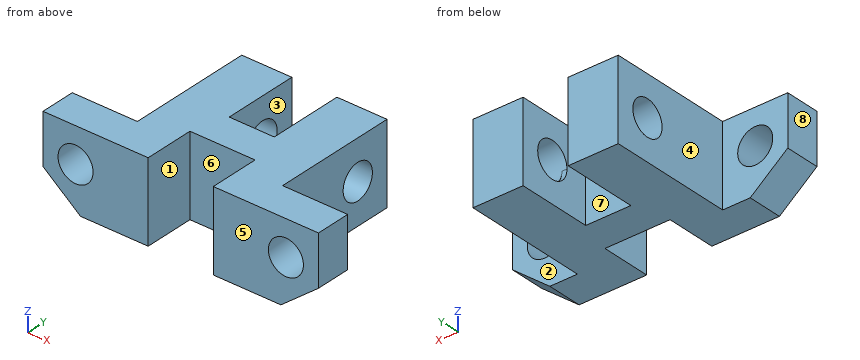
Autodesk Fusion 360 part; units mm, degrees
sketch "Boceto1" plane through (0, 0, 0) normal (0, 0, 1) x (1, 0, 0)
  line L0 (0, 0) -> (4.5, 0)
  line L1 (4.5, 0) -> (4.5, 15)
  line L2 (4.5, 15) -> (14.5, 15)
  line L3 (14.5, 15) -> (14.5, -10)
  line L4 (14.5, -10) -> (27.5, -10)
  line L5 (27.5, -10) -> (27.5, -17)
  line L6 (0, -7) -> (6.5, -7)
  line L7 (6.5, -7) -> (6.5, -17)
  line L8 (6.5, -17) -> (27.5, -17)
  line L9 (0, -7) -> (-6.5, -7)
  line L10 (-27.5, -10) -> (-27.5, -17)
  line L11 (-6.5, -7) -> (-6.5, -17)
  line L12 (-6.5, -17) -> (-27.5, -17)
  line L13 (-14.5, -10) -> (-27.5, -10)
  line L14 (-4.5, 0) -> (-4.5, 15)
  line L15 (-14.5, 15) -> (-14.5, -10)
  line L16 (0, 0) -> (-4.5, 0)
  line L17 (-4.5, 15) -> (-14.5, 15)
  dimension "d1" = 4.5
  dimension "d2" = 15
  dimension "d3" = 10
  dimension "d4" = 25
  dimension "d5" = 13
  dimension "d6" = 7
  dimension "d7" = 6.5
  dimension "d8" = 7
  dimension "d9" = 32
extrude "Extruir1" add sketch "Boceto1" along normal blind 16
sketch "Boceto2" plane through (0, 0, 0) normal (1, 0, 0) x (0, 1, 0)
  circle A0 centre (8, 8.0871) radius 3.5
  line L0 (15, 0) -> (15, 16)
  dimension "d12" = 7
  dimension "d13" = 7
sketch "Boceto3" plane through (-14.5, 0, 0) normal (-1, 0, 0) x (0, -1, 0)
  line L0 (-15, 0) -> (10, 0)
  line L1 (10, 0) -> (10, 16)
  line L2 (10, 16) -> (-15, 16)
  line L3 (-15, 16) -> (-15, 0)
  circle A0 centre (-8, 8) radius 3.5
  dimension "d14" = 7
extrude "Extruir2" cut sketch "Boceto2" along normal blind 20
extrude "Extruir3" cut sketch "Boceto3" against normal blind 20 contours A0
sketch "Boceto4" plane through (0, -10, 0) normal (0, 1, 0) x (-1, 0, 0)
  line L0 (-27.5, 0) -> (-14.5, 0)
  line L1 (-14.5, 0) -> (-14.5, 16)
  line L2 (-14.5, 16) -> (-27.5, 16)
  line L3 (-27.5, 16) -> (-27.5, 0)
  line L4 (-27.5, 0) -> (-20, 0)
  line L5 (-27.5, 6) -> (-27.5, 0)
  line L6 (-27.5, 6) -> (-20, 0)
extrude "Extruir4" cut sketch "Boceto4" against normal blind 8 contours L0 L3 L4 L5 L6
mirror "Simetría1" about plane through (0, 0, 0) normal (1, 0, 0) of "Extruir4"
sketch "Boceto5" plane through (0, -10, 0) normal (0, 1, 0) x (-1, 0, 0)
  line L0 (-27.5, 6) -> (-20, 0)
  line L1 (-20, 0) -> (-14.5, 0)
  line L2 (-14.5, 0) -> (-14.5, 16)
  line L3 (-14.5, 16) -> (-27.5, 16)
  line L4 (-27.5, 16) -> (-27.5, 6)
  circle A0 centre (-21, 9) radius 3.5
  dimension "d27" = 7
  dimension "d28" = 7
extrude "Extruir5" cut sketch "Boceto5" against normal blind 10 contours A0
mirror "Simetría2" about plane through (0, 0, 0) normal (1, 0, 0) of "Extruir5"
Verification items for the finished model (mm, model axes). Face numbers are marked on the shaded views. A direction names the side the tool comes from. Coordinates: 2 decimals unless noted, no trailing zeros. Loops run counter-clockwise (first coordinate to the right, second up) from the corner with the lowest first, then second, coordinate; pieces in that order, holes last. Notation, with made-up numbers: (62, 55.25) - (68, 55.25) arc R22 cw to (68, 75.25) - close; hole circle Ø8 at (-24, 61.25). An arc over 180 degrees is marked (long way). Put each result on its own line as item: value.
Item 1: Scan lines: line 1 along X through (y, z) = (1, 8.5); line 2 along X through (y, z) = (-7.5, 8.25); line 3 along X through (y, z) = (-2, 12.5). Record each from-to range of solid material in increasing order.
Conclusion:
line 1: x = -14.5 to -4.5, 4.5 to 14.5
line 2: x = -14.5 to -6.5, 6.5 to 14.5
line 3: x = -14.5 to 14.5
Item 2: Section check B-B (x = -21). Enter the section's corners in (y, z), then the cut area to 3 significant figures.
Conclusion:
outline: (-17, 0.8) - (-10, 0.8) - (-10, 5.5) - (-17, 5.5) - close; (-17, 12.5) - (-10, 12.5) - (-10, 16) - (-17, 16) - close
area: 57.4 mm2
Item 3: Gauge pin test, flat ends, axial feed: pin 1 Ø7.5 at (y, z) = (7.5, 10) entering from -X; pin 2 Ø4 at (y, z) = (8, 8) entering from +X; pin 3 Ø6 at (x, y) = (-7.5, -7) entering from -Z; pin 4 Ø2 at (x, z) = (-4.5, 7) entering from -Y. Record the tip position at first contact, or that the pin passes through.
Conclusion:
pin 1: stops at x = -14.5
pin 2: passes through
pin 3: stops at z = 0
pin 4: stops at y = -7
Item 4: Section check A-A (y = -11). Enter the section's corners in (x, z).
Conclusion:
outline: (-27.5, 6) - (-20, 0) - (-6.5, 0) - (-6.5, 16) - (-27.5, 16) - close; (6.5, 0) - (20, 0) - (27.5, 6) - (27.5, 16) - (6.5, 16) - close; hole circle Ø7 at (-21, 9); hole circle Ø7 at (21, 9)
Item 5: Set-up check for the marked faces 1, 2, 3 and 4: record each of +Z, -Z, +X, -X, +Y, -Y from which the full face is reachable in a straight line by a thin tool's end or side.
Conclusion:
face 1: +Z, -Z, -Y
face 2: +Z, -Z, +X, +Y
face 3: +Z, -Z, +Y
face 4: +Z, -Z, -X, +Y
Item 6: Draft check along X on the marked faces 5, 6, 7 and 8. Enter one of: pulls with the +X half, pulls with the -X half, needs draft (parallel to the pull), parting line crosses it, or undercut.
Conclusion:
face 5: needs draft
face 6: undercut
face 7: undercut
face 8: pulls with the -X half
Item 7: Section check D-D (y = 8). Enter the section's corners in (x, z), then the cut area to 3 significant figures.
Conclusion:
outline: (-14.5, 0) - (-4.5, 0) - (-4.5, 4.5) - (-14.5, 4.5) - close; (-14.5, 11.5) - (-4.5, 11.5) - (-4.5, 16) - (-14.5, 16) - close; (4.5, 0) - (14.5, 0) - (14.5, 4.59) - (5.5, 4.59) - (5.5, 4.5) - (4.5, 4.5) - close; (4.5, 11.59) - (14.5, 11.59) - (14.5, 16) - (4.5, 16) - close
area: 180 mm2
Item 8: Section check C-C (y = 2.5). Enter the section's corners in (x, z), then the cut area to 3 significant figures.
Conclusion:
outline: (-14.5, 0) - (-4.5, 0) - (-4.5, 16) - (-14.5, 16) - close; (4.5, 0) - (14.5, 0) - (14.5, 16) - (4.5, 16) - close
area: 320 mm2
